```python
from build123d import *

# Parameters (mm, degrees)
SKETCH_W        = 60.1
SKETCH_H        = 97.2
PAD_DEPTH       = 30
POCKET_DEPTH    = 2
SKETCH002_W     = 60.1
SKETCH002_H     = 97.2
SKETCH002_R     = 0.95
PAD001_DEPTH    = 3
SKETCH003_R     = 2.5
SKETCH003_R_2   = 0.95
PAD002_DEPTH    = 3
SKETCH004_R     = 6.5
POCKET001_DEPTH = 4.001
SKETCH005_R     = 1.25
POCKET002_DEPTH = 28.001


with BuildPart() as part:
    # Sketch → Pad (new body)
    with BuildSketch(Plane.XY):
        with BuildLine():
            Line((0, -9), (60.1, -9))
            ThreePointArc((60.1, -9), (66.463961, -6.363961), (69.1, 0))
            Line((69.1, 0), (69.1, 92.2))
            ThreePointArc((69.1, 92.2), (66.463961, 98.563961), (60.1, 101.2))
            Line((60.1, 101.2), (0, 101.2))
            ThreePointArc((0, 101.2), (-6.363961, 98.563961), (-9, 92.2))
            Line((-9, 92.2), (-9, 0))
            ThreePointArc((-9, 0), (-6.363961, -6.363961), (0, -9))
        make_face()
        with Locations((30.05, 48.6)):
            Rectangle(SKETCH_W, SKETCH_H, mode=Mode.SUBTRACT)
    extrude(amount=PAD_DEPTH)

    # Sketch001 (on Face14 of Pad) → Pocket (cut)
    with BuildSketch(Plane.XY.offset(30)):
        with BuildLine():
            Line((0, 98.7), (60.1, 98.7))
            ThreePointArc((66.6, 92.2), (64.696194, 96.796194), (60.1, 98.7))
            Line((66.6, 92.2), (66.6, 0))
            ThreePointArc((60.1, -6.5), (64.696194, -4.596194), (66.6, 0))
            Line((60.1, -6.5), (0, -6.5))
            ThreePointArc((-6.5, 0), (-4.596194, -4.596194), (0, -6.5))
            Line((-6.5, 0), (-6.5, 92.2))
            ThreePointArc((0, 98.7), (-4.596194, 96.796194), (-6.5, 92.2))
        make_face()
    extrude(amount=-POCKET_DEPTH, mode=Mode.SUBTRACT)

    # Sketch002 (on Face4 of Pocket) → Pad001 (join)
    with BuildSketch(Plane(origin=(0, 0, 0), x_dir=(1, 0, 0), z_dir=(0, 0, -1))):
        with Locations((30.05, -48.6)):
            Rectangle(SKETCH002_W, SKETCH002_H)
        with Locations((8.05, -79.2)):
            Circle(SKETCH002_R, mode=Mode.SUBTRACT)
        with Locations((30.05, -64.7)):
            Circle(SKETCH002_R, mode=Mode.SUBTRACT)
        with Locations((30.05, -93.7)):
            Circle(SKETCH002_R, mode=Mode.SUBTRACT)
    extrude(amount=-PAD001_DEPTH)

    # Sketch003 (on Face24 of Pad001) → Pad002 (join)
    with BuildSketch(Plane.XY.offset(3)):
        with Locations((8.05, 79.2)):
            Circle(SKETCH003_R)
        with Locations((8.05, 79.2)):
            Circle(SKETCH003_R_2, mode=Mode.SUBTRACT)
        with Locations((30.05, 93.7)):
            Circle(SKETCH003_R)
        with Locations((30.05, 93.7)):
            Circle(SKETCH003_R_2, mode=Mode.SUBTRACT)
        with Locations((30.05, 64.7)):
            Circle(SKETCH003_R)
        with Locations((30.05, 64.7)):
            Circle(SKETCH003_R_2, mode=Mode.SUBTRACT)
    extrude(amount=PAD002_DEPTH)

    # Sketch004 (on Face28 of Pad002) → Pocket001 (cut, through all)
    with BuildSketch(Plane.XZ.offset(-97.2)):
        with Locations((14.85, 14)):
            Circle(SKETCH004_R)
        with Locations((45.25, 14)):
            Circle(SKETCH004_R)
    extrude(amount=-POCKET001_DEPTH, mode=Mode.SUBTRACT)

    # Sketch005 (on Face25 of Pocket001) → Pocket002 (cut, through all)
    with BuildSketch(Plane.XY.offset(28)):
        with Locations((-3.35, 83.45)):
            Circle(SKETCH005_R)
        with Locations((-3.35, 8.45)):
            Circle(SKETCH005_R)
        with Locations((63.45, 83.45)):
            Circle(SKETCH005_R)
        with Locations((63.45, 8.45)):
            Circle(SKETCH005_R)
    extrude(amount=-POCKET002_DEPTH, mode=Mode.SUBTRACT)


solid = part.part
```
Source: CAD feature listing. Evaluate the final solid. Frame: model axes, mm. A direction names the side the tool comes from. Give positions to 0.01 mm unless a question says otherwise; leave off trailing zeros. Order: outer loops, then holes, each group sorted by start corner. A loop starts at its lowest first (then second) coordinate and runs counter-clockwise, first axis right, second up.
(1) Access query for faces 1 (the face through (8, 78, 6)), 2 (the face through (-2.678, 84.504, 14.196)). Directions: +Z, -Z, +X, -X, +Y, -Y. A direction counts if a zero-diameter tool reaches every point of the face in a straight line with its end or side. Return the directions, or none.
(2) Contact query for flat-ended pins moving along their axis: P1, Ø1.5, axis at x = 29.5, y = 64, coming from the +Z side; P2, Ø1.5, axis at x = 63.45, y = 83.45, coming from the +Z side; P3, Ø2, axis at x = 32.5, y = 43, coming from the +Z side. Output: stop coordinate, or through.
(3) Section query A-A (z = 14). Return the cut outline in (x, y), plus the area to 3 significant figures.
(4) Section query D-D (x = 63.5). Return the cut outline in (y, z).
(5) Material intervals for line 1 along Y through (x, z) = (30.05, 3.7); line 2 along Y through (x, z) = (8.05, 4.2); line 3 along Y through (x, z) = (16, 20.5), sorted ascending.
(6) Section query B-B (y = 8.45). Return the cut outline in (x, z), plus the area to 3 significant figures.
(7) Pull-direction query (X, two-part tool) for faces 3 (the face through (66.534, 98.494, 14.79)), 4 (the face through (18.344, 99.172, 19.481)), 5 (the face through (-9, 47, 15)); classes: +X half, -X half, draft (parallel to the pull), parting line (faces both ways), or undercut.
(8) Section query C-C (z = 26.5). Return the cut outline in (x, y).
Outcome:
1. face 1: +Z
1. face 2: +Z, -Z
2. P1: stops at z = 6
2. P2: passes through
2. P3: stops at z = 3
3. outline: (-9, 0) arc R9 ccw to (0, -9) - (60.1, -9) arc R9 ccw to (69.1, 0) - (69.1, 92.2) arc R9 ccw to (60.1, 101.2) - (51.75, 101.2) - (51.75, 97.2) - (60.1, 97.2) - (60.1, 0) - (0, 0) - (0, 97.2) - (8.35, 97.2) - (8.35, 101.2) - (0, 101.2) arc R9 ccw to (-9, 92.2) - close; (21.35, 97.2) - (38.75, 97.2) - (38.75, 101.2) - (21.35, 101.2) - close; hole circle Ø2.5 at (-3.35, 8.45); hole circle Ø2.5 at (-3.35, 83.45); hole circle Ø2.5 at (63.45, 8.45); hole circle Ø2.5 at (63.45, 83.45)
3. area: 2,570 mm2
4. outline: (-8.33, 0) - (7.2, 0) - (7.2, 28) - (-5.54, 28) - (-5.54, 30) - (-8.33, 30) - close; (9.7, 0) - (82.2, 0) - (82.2, 28) - (9.7, 28) - close; (84.7, 0) - (100.53, 0) - (100.53, 30) - (97.74, 30) - (97.74, 28) - (84.7, 28) - close
5. line 1: y = -9 to 0, 62.2 to 63.75, 65.65 to 67.2, 91.2 to 92.75, 94.65 to 96.2, 97.2 to 101.2
5. line 2: y = -9 to 0, 76.7 to 78.25, 80.15 to 81.7, 97.2 to 101.2
5. line 3: y = -9 to 0, 97.2 to 101.2
6. outline: (-9, 0) - (-4.6, 0) - (-4.6, 28) - (-6.5, 28) - (-6.5, 30) - (-9, 30) - close; (-2.1, 0) - (62.2, 0) - (62.2, 28) - (60.1, 28) - (60.1, 3) - (0, 3) - (0, 28) - (-2.1, 28) - close; (64.7, 0) - (69.1, 0) - (69.1, 30) - (66.6, 30) - (66.6, 28) - (64.7, 28) - close
6. area: 554 mm2
7. face 3: +X half
7. face 4: undercut
7. face 5: -X half
8. outline: (-9, 0) arc R9 ccw to (0, -9) - (60.1, -9) arc R9 ccw to (69.1, 0) - (69.1, 92.2) arc R9 ccw to (60.1, 101.2) - (0, 101.2) arc R9 ccw to (-9, 92.2) - close; hole circle Ø2.5 at (-3.35, 8.45); hole circle Ø2.5 at (-3.35, 83.45); hole (0, 0) - (60.1, 0) - (60.1, 97.2) - (0, 97.2) - close; hole circle Ø2.5 at (63.45, 8.45); hole circle Ø2.5 at (63.45, 83.45)
